Here's how the part is built. I have some questions about the finished solid (model axes, mm). Face numbers are marked on the shaded views. A direction names the side the tool comes from. Round coordinates to 2 decimals unless told otherwise and drop trailing zeros. Use a Markdown table: item, result.
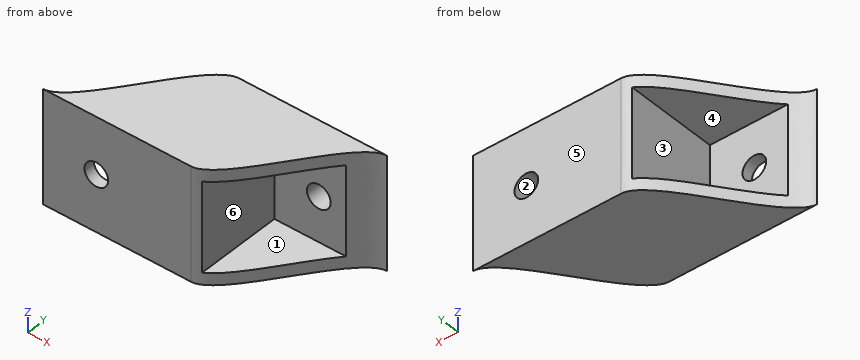
```python
from build123d import *

# Parameters (mm, degrees)
SKETCH1_W           = 86
SKETCH1_H           = 36
BOSS_EXTRUDE1_DEPTH = 38.2
CUT_EXTRUDE2_DEPTH  = 101.753362227
SKETCH3_R           = 4
CUT_EXTRUDE5_DEPTH  = 101.753362386
SKETCH3_9_R         = 4
CUT_EXTRUDE7_DEPTH  = 101.753362386
SKETCH6_W           = 33
SKETCH6_H           = 30.2
CUT_EXTRUDE8_DEPTH  = 32.2
CUT_EXTRUDE9_START  = -6
SKETCH6_8_W         = 33
SKETCH6_8_H         = 30.2
CUT_EXTRUDE9_DEPTH  = 95.753362386


with BuildPart() as part:
    # Sketch1 → Boss-Extrude1 (new body)
    with BuildSketch(Plane.XY):
        with Locations((43, 18)):
            Rectangle(SKETCH1_W, SKETCH1_H)
    extrude(amount=BOSS_EXTRUDE1_DEPTH)

    # Sketch2 → Cut-Extrude2 (cut, through all)
    with BuildSketch(Plane.XY):
        with BuildLine():
            Line((86, 36), (86, 0))
            Line((86, 0), (50, 0))
            add(Edge.make_bspline(
                [(50, 0), (60, 0), (76, 36), (86, 36)],
                knots=[0, 0, 0, 0, 1, 1, 1, 1], degree=3))
        make_face()
        with BuildLine():
            Line((36, 36), (0, 36))
            Line((0, 36), (0, 0))
            add(Edge.make_bspline(
                [(36, 36), (26, 36), (10, 0), (0, 0)],
                knots=[0, 0, 0, 0, 1, 1, 1, 1], degree=3))
        make_face()
    extrude(amount=CUT_EXTRUDE2_DEPTH, mode=Mode.SUBTRACT)

    # Sketch3 → Cut-Extrude5 (cut, through all)
    with BuildSketch(Plane(origin=(0, 0, 0), x_dir=(1, 0, 0), z_dir=(0, 1, 0))):
        with Locations(Location((18, -19.1, 0), (0, 0, 90))):
            Circle(SKETCH3_R)
    extrude(amount=CUT_EXTRUDE5_DEPTH, mode=Mode.SUBTRACT)

    # Sketch3_9 → Cut-Extrude7 (cut, through all)
    with BuildSketch(Plane(origin=(0, 0, 0), x_dir=(1, 0, 0), z_dir=(0, 1, 0))):
        with Locations(Location((68, -19.1, 0), (0, 0, 90))):
            Circle(SKETCH3_9_R)
    extrude(amount=CUT_EXTRUDE7_DEPTH, mode=Mode.SUBTRACT)

    # Sketch6 → Cut-Extrude8 (cut)
    with BuildSketch(Plane(origin=(0, 36, 0), x_dir=(1, 0, 0), z_dir=(0, 1, 0))):
        with Locations((16.5, -19.1)):
            Rectangle(SKETCH6_W, SKETCH6_H)
    extrude(amount=-CUT_EXTRUDE8_DEPTH, mode=Mode.SUBTRACT)

    # Sketch6_8 → Cut-Extrude9 (cut, through all)
    with BuildSketch(Plane(origin=(0, 36, 0), x_dir=(1, 0, 0), z_dir=(0, 1, 0)).offset(CUT_EXTRUDE9_START)):
        with Locations((69.5, -19.1)):
            Rectangle(SKETCH6_8_W, SKETCH6_8_H)
    extrude(amount=-CUT_EXTRUDE9_DEPTH, mode=Mode.SUBTRACT)


solid = part.part
```
Q1. We'd pull the mould along X, two halves only. Please class the marked faces 1, 2 and 3: pulls with the +X half, pulls with the -X half, needs draft (parallel to the pull), parting line crosses it, or undercut.
Return value:
| item | result |
|---|---|
| face 1 | needs draft |
| face 2 | undercut |
| face 3 | pulls with the -X half |
Q2. For the marked faces 4, 5 and 6, which set-ups out of +Z, -Z, +X, -X, +Y, -Y let a thin tool reach every point of the face, with its end or its side?
Return value:
| item | result |
|---|---|
| face 4 | -X, +Y |
| face 5 | +Z, -Z, +X, -X, +Y |
| face 6 | +X, -Y |
Q3. Will these pins go through, and if not, where does the flat tip stop? P1, Ø15, axis at y = 20.5, z = 14.5, coming from the -X side; P2, Ø2, axis at y = 5, z = 19, coming from the +X side; P3, Ø19.5, axis at x = 60, z = 23, coming from the -Y side.
Return value:
| item | result |
|---|---|
| P1 | stops at x = 33 |
| P2 | stops at x = 53 |
| P3 | stops at y = 0.01 |
Q4. I need wall thicknesses on line 1 (Z direction, x = 71, y = 27.5); line 2 (Z direction, x = 18, y = 1.3); line 3 (X direction, y = 6.5, z = 31). Which ranges of each line are inside material? Lowest first, please. Write a range as from..to.
Return value:
| item | result |
|---|---|
| line 1 | z = 0..4, 34.2..38.2 |
| line 2 | z = 0..15.1, 23.1..38.2 |
| line 3 | x = 33..53 |
Q5. Imagine slicing it at A-A, the plane z = 21.5. Give the number of separate pieces and of enclosed holes in the cut face, then the cut area to 3 significant figures.
Return value:
| item | result |
|---|---|
| separate pieces | 3 |
| enclosed holes | 0 |
| area | 929 mm^2 |
